```python
from build123d import *

# Parameters (mm, degrees)
EXTRUDE_1_DEPTH     = 80
SKETCH_3_R          = 5
CUT_EXTRUDE_1_DEPTH = 10


with BuildPart() as part:
    # Эскиз2 → Вытянуть-Тонкостенный1 (new body)
    with BuildSketch(Plane(origin=(0, 0, 0), x_dir=(1, 0, 0), z_dir=(0, 1, 0))):
        Polygon((0, 42), (0, 0), (10, 0), (10, 2), (2, 2), (2, 42), align=None)
    extrude(amount=EXTRUDE_1_DEPTH)

    # Эскиз3 → Вырез-Вытянуть1 (cut)
    with BuildSketch(Plane.ZY):
        with Locations((-22, 40)):
            Circle(SKETCH_3_R)
    extrude(amount=-CUT_EXTRUDE_1_DEPTH, mode=Mode.SUBTRACT)


solid = part.part
```
Verification items for the finished model (mm, model axes). A direction names the side the tool comes from. Round coordinates to 2 decimals unless told otherwise and drop trailing zeros. Order: outer loops, then holes, each group sorted by start corner. A loop starts at its lowest first (then second) coordinate and runs counter-clockwise, first axis right, second up. Notation, with made-up numbers: (-1, -32.75) -> (46, -32.75) arc R33 cw to (46, 1.25) -> close; hole circle Ø4 at (23, -33). An arc over 180 degrees is marked (long way). Put each result on its own line as item: value. Start each with the question number.
(1) Material ranges on line 1 along Y through (x, z) = (0.5, -22); line 2 along Z through (x, y) = (5, 58); line 3 along X through (y, z) = (30.5, -8.5), recorded low to high.
(2) Section check C-C (x = 1). Enter the section's corners in (y, z), then the cut area to 3 significant figures.
(3) Draft check along Z on faces 1 (the face through (5, 39, 0)), 2 (the face through (6, 39, -2)), 3 (the face through (1.6, 0, -18)), 4 (the face through (0.986, 44.957, -22.651)). Enter one of: +Z half, -Z half, draft (parallel to the pull), parting line (faces both ways), or undercut.
(4) Tool access check on faces 5 (the face through (1, 39, -42)), 6 (the face through (2, 39, -31)). Record the directions out of +Z, -Z, +X, -X, +Y, -Y that give a thin tool (end or side, any length) a straight path to the whole face; none if there is none.
(5) Section check A-A (y = 40). Enter the section's corners in (x, z), then the cut area to 3 significant figures.
(6) Section check D-D (y = 74). Enter the section's corners in (x, z), then the cut area to 3 significant figures.
(7) Depth check by flat-ended pin: pin 1 Ø4 at (x, z) = (1, -23) entering from -Y; pin 2 Ø6 at (x, y) = (7.5, 11.5) entering from -Z; pin 3 Ø13 at (y, z) = (40, -22) entering from +X. Enter the tip coordinate at first touch or a pass-through.
(8) Section check B-B (z = -22). Enter the section's corners in (x, y).
Completed:
1. line 1: y = 0 to 35, 45 to 80
1. line 2: z = -2 to 0
1. line 3: x = 0 to 2
2. outline: (0, -42) -> (80, -42) -> (80, 0) -> (0, 0) -> close; hole circle Ø10 at (40, -22)
2. area: 3,280 mm2
3. face 1: +Z half
3. face 2: -Z half
3. face 3: draft
3. face 4: undercut
4. face 5: -Z, +X, -X, +Y, -Y
4. face 6: -Z, +X, +Y, -Y
5. outline: (0, -42) -> (2, -42) -> (2, -27) -> (0, -27) -> close; (0, -17) -> (2, -17) -> (2, -2) -> (10, -2) -> (10, 0) -> (0, 0) -> close
5. area: 80.0 mm2
6. outline: (0, -42) -> (2, -42) -> (2, -2) -> (10, -2) -> (10, 0) -> (0, 0) -> close
6. area: 100 mm2
7. pin 1: stops at y = 0
7. pin 2: stops at z = -2
7. pin 3: stops at x = 2
8. outline: (0, 0) -> (2, 0) -> (2, 35) -> (0, 35) -> close; (0, 45) -> (2, 45) -> (2, 80) -> (0, 80) -> close
